```python
from build123d import *

# Parameters (mm, degrees)
SKETCH1_W               = 30
SKETCH1_H               = 30
MAIN_BODY_DEPTH         = 11
SKETCH2_W               = 17.84
SKETCH2_H               = 2.8
WIRE_HOLE_DEPTH         = 6
BOARD_CAVITY_DEPTH      = 3
BOARD_CAVITY_DEPTH_BACK = 17.2
SKETCH3_W               = 20.5
SKETCH3_H               = 3.6
SKETCH4_W               = 10
SKETCH4_H               = 10
LIGHT_BOX_DEPTH         = 2
SKETCH5_R               = 2.5
CUT_EXTRUDE4_DEPTH      = 5
SKETCH7_W               = 20.5
SKETCH7_H               = 3.6
CUT_EXTRUDE5_DEPTH      = 1
BOSS_EXTRUDE1_DEPTH     = 30
BOSS_EXTRUDE2_START     = 2
SKETCH11_W              = 10
SKETCH11_H              = 10
SKETCH11_R              = 2.5
BOSS_EXTRUDE2_DEPTH     = 2
SKETCH12_W              = 44.564275197
SKETCH12_H              = 6
CUT_EXTRUDE6_DEPTH      = 40
FILLET2_R               = 1


with BuildPart() as part:
    # Sketch1 → Main Body (new body)
    with BuildSketch(Plane(origin=(0, 0, 0), x_dir=(1, 0, 0), z_dir=(0, 1, 0))):
        Rectangle(SKETCH1_W, SKETCH1_H)
    extrude(amount=MAIN_BODY_DEPTH)

    # Sketch2 → Wire Hole (cut)
    with BuildSketch(Plane.XZ):
        with Locations((0, 8.6)):
            Rectangle(SKETCH2_W, SKETCH2_H)
    extrude(amount=-WIRE_HOLE_DEPTH, mode=Mode.SUBTRACT)

    # Sketch3 → Board Cavity (cut, two sides: drawn at the far end of the back side and taken through both)
    with BuildSketch(Plane.XY.offset(7.2).offset(-BOARD_CAVITY_DEPTH_BACK)):
        with Locations((0, 4.2)):
            Rectangle(SKETCH3_W, SKETCH3_H)
    extrude(amount=BOARD_CAVITY_DEPTH + BOARD_CAVITY_DEPTH_BACK, mode=Mode.SUBTRACT)

    # Sketch4 → Light Box (cut)
    with BuildSketch(Plane.XZ.offset(-6)):
        with Locations((0, 0.05)):
            Rectangle(SKETCH4_W, SKETCH4_H)
    extrude(amount=-LIGHT_BOX_DEPTH, mode=Mode.SUBTRACT)

    # Sketch5 → Cut-Extrude4 (cut)
    with BuildSketch(Plane.XZ.offset(-8)):
        with Locations(Location((0, 0, 0), (0, 0, 270))):
            Circle(SKETCH5_R)
    extrude(amount=-CUT_EXTRUDE4_DEPTH, mode=Mode.SUBTRACT)

    # Sketch7 → Cut-Extrude5 (cut)
    with BuildSketch(Plane.XY.offset(-10)):
        with Locations((0, 4.2)):
            Rectangle(SKETCH7_W, SKETCH7_H)
    extrude(amount=-CUT_EXTRUDE5_DEPTH, mode=Mode.SUBTRACT)

    # Sketch8 → Boss-Extrude1 (add)
    with BuildSketch(Plane(origin=(0, 0, -15), x_dir=(-1, 0, 0), z_dir=(0, 0, -1))):
        Polygon((-15, 5.5), (-15, 3.8), (-17.2, 3.8), (-17.2, 2.5), (-19.75, 2.5), (-19.75, 8.5), (-17.2, 8.5), (-17.2, 7.2), (-15, 7.2), align=None)
    boss_extrude1 = extrude(amount=-BOSS_EXTRUDE1_DEPTH)

    # Mirror1: Boss-Extrude1 across plane
    add(boss_extrude1.mirror(Plane(origin=(0, 0, 0), x_dir=(0, 0, 1), z_dir=(1, 0, 0))))

    # Sketch9 → Cut-Revolve6 (revolve, cut)
    with BuildSketch(Plane.XY, mode=Mode.PRIVATE) as cut_revolve6_sk:
        with BuildLine():
            Line((-0.715, 25.989433281), (-0.715, 8))
            Line((-0.715, 8), (-1.3, 8))
            ThreePointArc((-1.3, 8), (-9.90524506, 17.284063213), (-0.715, 25.989433281))
        make_face()
    revolve(cut_revolve6_sk.sketch.rotate(Axis((0, 0, 0), (0, -1, 0)), 90), axis=Axis((0, 0, 0), (0, -1, 0)), mode=Mode.SUBTRACT)

    # Sketch11 → Boss-Extrude2 (add)
    with BuildSketch(Plane.XZ.offset(-8).offset(BOSS_EXTRUDE2_START)):
        with Locations((0, 0.05)):
            Rectangle(SKETCH11_W, SKETCH11_H)
        with Locations(Location((0, 0, 0), (0, 0, 270))):
            Circle(SKETCH11_R, mode=Mode.SUBTRACT)
    extrude(amount=-BOSS_EXTRUDE2_DEPTH)

    # Sketch12 → Cut-Extrude6 (cut)
    with BuildSketch(Plane(origin=(0, 0, -15), x_dir=(-1, 0, 0), z_dir=(0, 0, -1))):
        with Locations((-0.667629591, 3)):
            Rectangle(SKETCH12_W, SKETCH12_H)
    extrude(amount=-CUT_EXTRUDE6_DEPTH, mode=Mode.SUBTRACT)

    # Fillet1: read off the stored shape, not the designer's step
    # Fillet1 outline → Fillet1 (revolve, cut)
    with BuildSketch(Plane.XY):
        with BuildLine():
            Line((6.484202234, 11), (6.484202234, 9.925552153))
            ThreePointArc((6.484202234, 9.925552153), (7.942042689, 10.72375702), (9.580981253, 11))
            Line((9.580981253, 11), (6.484202234, 11))
        make_face()
    revolve(axis=Axis((0, 0, 0), (0, 1, 0)), mode=Mode.SUBTRACT)

    # Fillet2
    fillet2_edges = [part.edges().sort_by_distance(p)[0] for p in [
        (-1e-09, 8.133109373, 2.499999999),
    ]]
    fillet(fillet2_edges, radius=FILLET2_R)

    # Sketch13 → Cut-Revolve7 (revolve, cut)
    with BuildSketch(Plane.XY, mode=Mode.PRIVATE) as cut_revolve7_sk:
        Polygon((-2.5, 7.332772815), (-3.832772815, 6), (0, 6), (0, 7.332772815), align=None)
    revolve(cut_revolve7_sk.sketch.rotate(Axis((0, 0, 0), (0, -1, 0)), 270), axis=Axis((0, 0, 0), (0, -1, 0)), mode=Mode.SUBTRACT)


solid = part.part
```
Input: part model. Units: mm. Frame: model coordinates. A direction names the side the tool comes from. Coordinates: 2 decimals unless noted, no trailing zeros. Write each loop counter-clockwise with the first axis right and the second up, starting at its lowest first coordinate (ties: lowest second). Pieces come first, ordered by that corner, then holes.
1) Material intervals for line 1 along X through (y, z) = (8.25, 4.75); line 2 along X through (y, z) = (8.9, 9); line 3 along X through (y, z) = (10.3, 2.5), sorted ascending.
2) Set-up query: faces 1 (the flat face through (-7, 11, -7)), 2 (the flat face through (16, 7.2, 0)), 3 (the flat face through (18, 8.5, 0)). Return all of +Z, -Z, +X, -X, +Y, -Y with unobstructed straight access to the full face (end or side cutting, diameter ignored); none if empty.
3) Section B-B on y = 10.45. Output: boundary loops of the cut face in (x, z).
4) Section A-A on z = 13.25. Output: boundary loops of the cut face in (x, y).
5) Pin query (flat end, axial travel): pin 1 Ø1.8 at (x, z) = (16, -5.5) entering from +Y; pin 2 Ø1.3 at (x, z) = (18, -1) entering from +Y. Return the tip coordinate at first contact, or that it passes through.
6) Mould query, pull axis X, two halves, no side actions, for faces 4 (the flat face through (-18, 8.5, 0)), 5 (the flat face through (-15, 9, 0)), 6 (the flat face through (-19.75, 7, 0)). Classes: pulls with the +X half, pulls with the -X half, needs draft (parallel to the pull), parting line crosses it, or undercut.
Check result:
1. line 1: x = -19.75 to -17.2, -15 to 15, 17.2 to 19.75
1. line 2: x = -15 to 15
1. line 3: x = -15 to -6.57, 6.57 to 15
2. face 1: +Z, -Z, +X, -X, +Y
2. face 2: +Z, -Z, +Y
2. face 3: +Z, -Z, +X, +Y
3. outline: (-15, -15) - (15, -15) - (15, 15) - (-15, 15) - close; hole circle Ø14.6 at (0, 0)
4. outline: (-19.75, 6) - (19.75, 6) - (19.75, 8.5) - (17.2, 8.5) - (17.2, 7.2) - (15, 7.2) - (15, 11) - (-15, 11) - (-15, 7.2) - (-17.2, 7.2) - (-17.2, 8.5) - (-19.75, 8.5) - close
5. pin 1: stops at y = 7.2
5. pin 2: stops at y = 8.5
6. face 4: needs draft
6. face 5: undercut
6. face 6: pulls with the -X half
